Check sheet for the modelled part. Datum: model origin and axes. Units: mm. Face numbers are marked on the shaded views. A direction names the side the tool comes from. Round coordinates to 2 decimals unless told otherwise and drop trailing zeros. Write each loop counter-clockwise with the first axis right and the second up, starting at its lowest first coordinate (ties: lowest second). Pieces come first, ordered by that corner, then holes. Notation, with made-up numbers: (36.5, -3.75) -> (80.5, -3.75) arc R12 cw to (80.5, 8.25) -> close; hole circle Ø2 at (56.25, -20). An arc over 180 degrees is marked (long way). One line per item, written item: value.
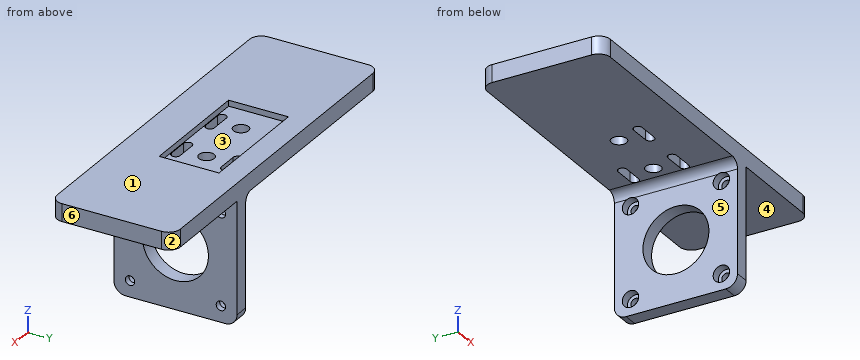
from build123d import *

# Parameters (mm, degrees)
SKETCH1_R               = 2.6
BOSS_EXTRUDE1_DEPTH     = 6
SKETCH8_W               = 40.4
SKETCH8_H               = 20.4
CUT_EXTRUDE4_DEPTH      = 2
SKETCH9_W               = 5
SKETCH9_H               = 42
BOSS_EXTRUDE2_DEPTH     = 42
FILLET1_R               = 4
FILLET2_R               = 3
SKETCH10_R              = 11.25
SKETCH10_R_2            = 1.6
CUT_EXTRUDE5_DEPTH      = 42
CUT_EXTRUDE6_DEPTH      = 3
CUT_EXTRUDE6_DEPTH_BACK = 3
SKETCH11_R              = 2.8


with BuildPart() as part:
    # Sketch1 → Boss-Extrude1 (new body)
    with BuildSketch(Plane.XY):
        with BuildLine():
            Line((-56, -1.5), (20, -1.5))
            Line((20, -1.5), (56, -1.5))
            ThreePointArc((56, -1.5), (58.828427125, -0.328427125), (60, 2.5))
            Line((60, 2.5), (60, 36.5))
            ThreePointArc((60, 36.5), (58.828427125, 39.328427125), (56, 40.5))
            Line((56, 40.5), (-56, 40.5))
            ThreePointArc((-56, 40.5), (-58.828427125, 39.328427125), (-60, 36.5))
            Line((-60, 36.5), (-60, 2.5))
            ThreePointArc((-60, 2.5), (-58.828427125, -0.328427125), (-56, -1.5))
        make_face()
        with Locations((10, 22.5)):
            Circle(SKETCH1_R, mode=Mode.SUBTRACT)
        with Locations((-10, 22.5)):
            Circle(SKETCH1_R, mode=Mode.SUBTRACT)
        with BuildLine():
            Line((-13.5, 15.5), (-6.5, 15.5))
            ThreePointArc((-6.5, 15.5), (-5, 14), (-6.5, 12.5))
            Line((-6.5, 12.5), (-13.5, 12.5))
            ThreePointArc((-13.5, 12.5), (-15, 14), (-13.5, 15.5))
        make_face(mode=Mode.SUBTRACT)
        with BuildLine():
            Line((13.5, 15.5), (6.5, 15.5))
            ThreePointArc((6.5, 15.5), (5, 14), (6.5, 12.5))
            Line((6.5, 12.5), (13.5, 12.5))
            ThreePointArc((13.5, 12.5), (15, 14), (13.5, 15.5))
        make_face(mode=Mode.SUBTRACT)
        with BuildLine():
            Line((13.5, 29.5), (6.5, 29.5))
            ThreePointArc((6.5, 29.5), (5, 31), (6.5, 32.5))
            Line((6.5, 32.5), (13.5, 32.5))
            ThreePointArc((13.5, 32.5), (15, 31), (13.5, 29.5))
        make_face(mode=Mode.SUBTRACT)
    extrude(amount=BOSS_EXTRUDE1_DEPTH)

    # Sketch8 → Cut-Extrude4 (cut)
    with BuildSketch(Plane.XY.offset(6)):
        with Locations((0, 22.5)):
            Rectangle(SKETCH8_W, SKETCH8_H)
    extrude(amount=-CUT_EXTRUDE4_DEPTH, mode=Mode.SUBTRACT)

    # Sketch9 → Boss-Extrude2 (add)
    with BuildSketch(Plane(origin=(0, 0, 0), x_dir=(-1, 0, 0), z_dir=(0, 0, -1))):
        with Locations((-20.5, 19.5)):
            Rectangle(SKETCH9_W, SKETCH9_H)
    extrude(amount=BOSS_EXTRUDE2_DEPTH)

    # Fillet1
    fillet1_edges = [part.edges().sort_by_distance(p)[0] for p in [
        (20.5, 40.5, -42),
        (20.5, -1.5, -42),
    ]]
    fillet(fillet1_edges, radius=FILLET1_R)

    # Fillet2
    fillet2_edges = [part.edges().sort_by_distance(p)[0] for p in [
        (18, 19.5, 0),
    ]]
    fillet(fillet2_edges, radius=FILLET2_R - 0.0001)  # a hair under: the kernel refuses the full size

    # Sketch10 → Cut-Extrude5 (cut)
    with BuildSketch(Plane(origin=(23, 0, 0), x_dir=(0, 0, -1), z_dir=(1, 0, 0))):
        with Locations(Location((21, 19.5, 0), (0, 0, 90))):
            Circle(SKETCH10_R)
        with Locations(Location((5.5, 35, 0), (0, 0, 90))):
            Circle(SKETCH10_R_2)
        with Locations(Location((36.5, 35, 0), (0, 0, 90))):
            Circle(SKETCH10_R_2)
        with Locations(Location((36.5, 4, 0), (0, 0, 90))):
            Circle(SKETCH10_R_2)
        with Locations(Location((5.5, 4, 0), (0, 0, 90))):
            Circle(SKETCH10_R_2)
    extrude(amount=-CUT_EXTRUDE5_DEPTH, mode=Mode.SUBTRACT)

    # Sketch11 → Cut-Extrude6 (cut, two sides: drawn at the far end of the back side and taken through both)
    with BuildSketch(Plane.ZY.offset(-18).offset(-CUT_EXTRUDE6_DEPTH_BACK)):
        with Locations(Location((-36.5, 35, 0), (0, 0, 180))):
            Circle(SKETCH11_R)
        with Locations(Location((-5.5, 35, 0), (0, 0, 26.765500577))):
            Circle(SKETCH11_R)
        with Locations(Location((-5.5, 4, 0), (0, 0, 26.765500577))):
            Circle(SKETCH11_R)
        with Locations(Location((-36.5, 4, 0), (0, 0, 180))):
            Circle(SKETCH11_R)
    extrude(amount=CUT_EXTRUDE6_DEPTH + CUT_EXTRUDE6_DEPTH_BACK, mode=Mode.SUBTRACT)


solid = part.part
Item 1: Mould release check, pull along Y, two halves, no side actions. Record for the marked faces 1, 2 and 3: pulls with the +Y half, pulls with the -Y half, needs draft (parallel to the pull), parting line crosses it, or undercut.
Answer:
face 1: needs draft
face 2: pulls with the +Y half
face 3: undercut
Item 2: Tool access check on the marked faces 4, 5 and 6. Record the directions out of +Z, -Z, +X, -X, +Y, -Y that give a thin tool (end or side, any length) a straight path to the whole face; none if there is none.
Answer:
face 4: -Z, +X, +Y, -Y
face 5: -Z, -X, +Y, -Y
face 6: +Z, -Z, +X, +Y, -Y
Item 3: Thickness scan on line 1 (Y direction, x = 19.8, z = -5.5); line 2 (Y direction, x = -10, z = 2); line 3 (Z direction, x = 19.7, y = 4). Record the ranges inside material, lowest first.
Answer:
line 1: y = -1.5 to 1.2, 6.8 to 32.2, 37.8 to 40.5
line 2: y = -1.5 to 12.5, 15.5 to 19.9, 25.1 to 40.5
line 3: z = -42 to -39.3, -33.7 to -8.3, -2.7 to 6
Item 4: Sectioned sample at A-A on x = 10. Enter the section's corners in (y, z).
Answer:
outline: (-1.5, 0) -> (12.5, 0) -> (12.5, 4) -> (12.3, 4) -> (12.3, 6) -> (-1.5, 6) -> close; (15.5, 0) -> (19.9, 0) -> (19.9, 4) -> (15.5, 4) -> close; (25.1, 0) -> (29.5, 0) -> (29.5, 4) -> (25.1, 4) -> close; (32.5, 0) -> (40.5, 0) -> (40.5, 6) -> (32.7, 6) -> (32.7, 4) -> (32.5, 4) -> close
Item 5: Sectioned sample at C-C on z = 2.5. Enter the section's corners in (x, y).
Answer:
outline: (-60, 2.5) arc R4 ccw to (-56, -1.5) -> (56, -1.5) arc R4 ccw to (60, 2.5) -> (60, 36.5) arc R4 ccw to (56, 40.5) -> (-56, 40.5) arc R4 ccw to (-60, 36.5) -> close; hole (-13.5, 12.5) -> (-6.5, 12.5) arc R1.5 ccw to (-6.5, 15.5) -> (-13.5, 15.5) arc R1.5 ccw to start; hole circle Ø5.2 at (-10, 22.5); hole (6.5, 12.5) -> (13.5, 12.5) arc R1.5 ccw to (13.5, 15.5) -> (6.5, 15.5) arc R1.5 ccw to start; hole (6.5, 29.5) -> (13.5, 29.5) arc R1.5 ccw to (13.5, 32.5) -> (6.5, 32.5) arc R1.5 ccw to start; hole circle Ø5.2 at (10, 22.5)
Item 6: Depth check by flat-ended pin: P1, Ø7, axis at x = -10, y = 22.5, coming from the -Z side; P2, Ø6, axis at y = 36, z = -37, coming from the -X side; P3, Ø3.5, axis at y = 35, z = -36.5, coming from the -X side; P4, Ø6, axis at y = 13.5, z = -21.5, coming from the +X side. Enter the tip coordinate at first touch or a pass-through.
Answer:
P1: stops at z = 0
P2: stops at x = 18
P3: stops at x = 21
P4: passes through
Item 7: Sectioned sample at B-B on z = -36.5. Enter the section's corners in (x, y), and give its area (3 significant figures).
Answer:
outline: (18, -1.5) -> (23, -1.5) -> (23, 2.4) -> (21, 2.4) -> (21, 1.2) -> (18, 1.2) -> close; (18, 6.8) -> (21, 6.8) -> (21, 5.6) -> (23, 5.6) -> (23, 33.4) -> (21, 33.4) -> (21, 32.2) -> (18, 32.2) -> close; (18, 37.8) -> (21, 37.8) -> (21, 36.6) -> (23, 36.6) -> (23, 40.5) -> (18, 40.5) -> close
area: 164 mm^2
Item 8: Sectioned sample at D-D on y = 27. Enter the section's corners in (x, z), and give its area (3 significant figures).
Answer:
outline: (-60, 0) -> (15, 0) arc R3 cw to (18, -3) -> (18, -12.61) -> (23, -12.61) -> (23, 0) -> (60, 0) -> (60, 6) -> (20.2, 6) -> (20.2, 4) -> (-20.2, 4) -> (-20.2, 6) -> (-60, 6) -> close; (18, -42) -> (23, -42) -> (23, -29.39) -> (18, -29.39) -> close
area: 767 mm^2
